Input: part model. Units: mm. Frame: model coordinates. Face numbers are marked on the shaded views. A direction names the side the tool comes from. Coordinates: 2 decimals unless noted, no trailing zeros. Order: outer loops, then holes, each group sorted by start corner. A loop starts at its lowest first (then second) coordinate and runs counter-clockwise, first axis right, second up. Notation, with made-up numbers: (73, 36) - (116, 36) arc R25 cw to (116, 70) - close; hole circle Ø2 at (-7, 79). An arc over 180 degrees is marked (long way). One line per question, with ' | ' between items.
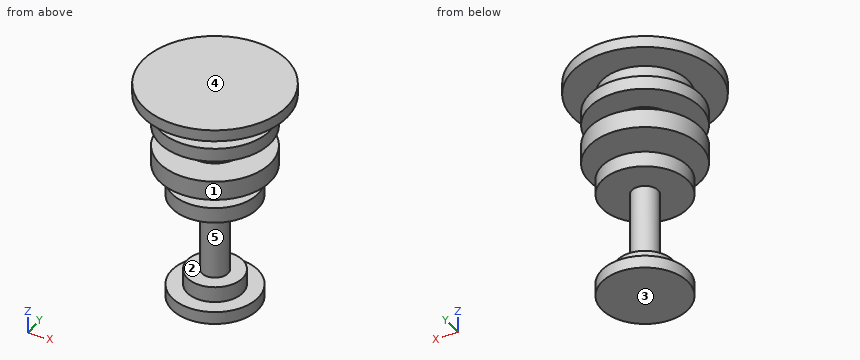
from build123d import *

# Parameters (mm, degrees)
F0_W   = 11.8117174134
F0_H   = 5.2878893912
F0_W_2 = 7.6244240627
F0_H_2 = 5.8166831732
F0_W_3 = 3.6154794507
F0_H_3 = 4.7591030598
F0_H_4 = 21.6046236455


with BuildPart() as f1:
    # F0 (on Front) → F1 (revolve)
    with BuildSketch(Plane.XZ):
        Polygon((0, 50.6880395114), (0, 53.8607798517), (-19.743559882, 53.8607798517), (-19.743559882, 50.6880395114), (-11.8117174134, 50.6880395114), align=None)
        with Locations((-5.9058587067, 48.0440948159)):
            Rectangle(F0_W, F0_H)
        Polygon((0, 41.6986197233), (0, 45.4001501203), (-11.8117174134, 45.4001501203), (-15.2488481253, 45.4001501203), (-15.2488481253, 41.6986197233), (-7.6244240627, 41.6986197233), align=None)
        with Locations((-3.8122120313, 38.7902781367)):
            Rectangle(F0_W_2, F0_H_2)
        Polygon((0, 30.594041571), (0, 35.8819365501), (-7.6244240627, 35.8819365501), (-15.2488481253, 35.8819365501), (-15.2488481253, 30.594041571), (-3.6154794507, 30.594041571), align=None)
        with Locations((-1.8077397253, 28.2144900411)):
            Rectangle(F0_W_3, F0_H_3)
        Polygon((0, 21.6046236455), (0, 25.8349385113), (-3.6154794507, 25.8349385113), (-11.8117174134, 25.8349385113), (-11.8117174134, 21.6046236455), (-3.6154794507, 21.6046236455), align=None)
        with Locations((-1.8077397253, 10.8023118228)):
            Rectangle(F0_W_3, F0_H_4)
        Polygon((0, -4.3060597964), (0, 0), (-3.6154794507, 0), (-7.6244240627, 0), (-7.6244240627, -4.3060597964), align=None)
        Polygon((0, -7.7431914397), (0, -4.3060597964), (-7.6244240627, -4.3060597964), (-11.8117174134, -4.3060597964), (-11.8117174134, -7.7431914397), align=None)
    revolve(axis=Axis((0, 0, 10.8023118228), (0, 0, -1)))


solid = f1.part
Item 1: Section C-C on z = 37. Return the cut outline in (x, y).
Data:
outline: circle Ø15.25 at (0, 0)
Item 2: Contact query for flat-ended pins moving along their axis: P1, Ø4, axis at x = 7.5, z = 41, coming from the +Y side; P2, Ø12, axis at x = 2.5, z = 10.5, coming from the -Y side; P3, Ø1.5, axis at y = 3.5, z = 20.5, coming from the -X side. Output: stop coordinate, or through.
Data:
P1: y = 14.17 | P2: y = -3.62 | P3: x = -2.35
Item 3: Ray query, line 1 (Z direction, x = 8, y = 4.5); line 2 (Z direction, x = 8.5, y = 10); line 3 (Z direction, x = 17, y = -2). Return the intervals inside material, ascending.
Data:
line 1: -7.74 to -4.31, 21.6 to 25.83, 30.59 to 35.88, 41.7 to 53.86 | line 2: 30.59 to 35.88, 41.7 to 45.4, 50.69 to 53.86 | line 3: 50.69 to 53.86
Item 4: Section A-A on x = 13. Return the cut outline in (y, z).
Data:
outline: (-14.86, 50.69) - (14.86, 50.69) - (14.86, 53.86) - (-14.86, 53.86) - close; (-7.97, 30.59) - (7.97, 30.59) - (7.97, 35.88) - (-7.97, 35.88) - close; (-7.97, 41.7) - (7.97, 41.7) - (7.97, 45.4) - (-7.97, 45.4) - close
Item 5: Section B-B on y = 8.5. Return the cut outline in (x, z).
Data:
outline: (-17.82, 50.69) - (-8.2, 50.69) - (-8.2, 45.4) - (-12.66, 45.4) - (-12.66, 41.7) - (12.66, 41.7) - (12.66, 45.4) - (8.2, 45.4) - (8.2, 50.69) - (17.82, 50.69) - (17.82, 53.86) - (-17.82, 53.86) - close; (-12.66, 30.59) - (12.66, 30.59) - (12.66, 35.88) - (-12.66, 35.88) - close; (-8.2, -7.74) - (8.2, -7.74) - (8.2, -4.31) - (-8.2, -4.31) - close; (-8.2, 21.6) - (8.2, 21.6) - (8.2, 25.83) - (-8.2, 25.83) - close
Item 6: Draft query along Z for the marked faces 1, 2 and 3. Return one class per face: released by +Z, released by -Z, zero draft, split by the parting line, or undercut.
Data:
face 1: zero draft | face 2: undercut | face 3: released by -Z
Item 7: Access query for the marked faces 4 and 5. Directions: +Z, -Z, +X, -X, +Y, -Y. A direction counts if a zero-diameter tool reaches every point of the face in a straight line with its end or side. Return the directions, or none.
Data:
face 4: +Z, +X, -X, +Y, -Y | face 5: none
